from build123d import *

# Parameters (mm, degrees)
SKETCH1_R           = 100
BOSS_EXTRUDE1_DEPTH = 325
SKETCH2_R           = 181.25545507
SKETCH2_R_2         = 10
BOSS_EXTRUDE2_DEPTH = 5
FILLET1_R           = 20
BOSS_EXTRUDE3_DEPTH = 5


with BuildPart() as part:
    # Sketch1 → Boss-Extrude1 (new, symmetric)
    with BuildSketch(Plane(origin=(0, 0, 0), x_dir=(1, 0, 0), z_dir=(0, 1, 0))):
        with Locations(Location((0, 0, 0), (0, 0, 270))):
            Circle(SKETCH1_R)
    extrude(amount=BOSS_EXTRUDE1_DEPTH, both=True)

    # Sketch2 → Boss-Extrude2 (add, symmetric)
    with BuildSketch(Plane.XZ.offset(325)):
        with Locations(Location((0, 0, 0), (0, 0, 270))):
            Circle(SKETCH2_R)
        with Locations(Location((0, 147.291814794, 0), (0, 0, 270))):
            Circle(SKETCH2_R_2, mode=Mode.SUBTRACT)
        with Locations(Location((127.558453381, 73.645907397, 0), (0, 0, 270))):
            Circle(SKETCH2_R_2, mode=Mode.SUBTRACT)
        with Locations(Location((127.558453381, -73.645907397, 0), (0, 0, 270))):
            Circle(SKETCH2_R_2, mode=Mode.SUBTRACT)
        with Locations(Location((0, -147.291814794, 0), (0, 0, 270))):
            Circle(SKETCH2_R_2, mode=Mode.SUBTRACT)
        with Locations(Location((-127.558453381, -73.645907397, 0), (0, 0, 270))):
            Circle(SKETCH2_R_2, mode=Mode.SUBTRACT)
        with Locations(Location((-127.558453381, 73.645907397, 0), (0, 0, 270))):
            Circle(SKETCH2_R_2, mode=Mode.SUBTRACT)
    extrude(amount=BOSS_EXTRUDE2_DEPTH, both=True)

    # Fillet1
    fillet1_edges = [part.edges().sort_by_distance(p)[0] for p in [
        (0, -320, -100),
    ]]
    fillet(fillet1_edges, radius=FILLET1_R)

    # Sketch3 → Boss-Extrude3 (add, symmetric)
    with BuildSketch(Plane(origin=(0, 325, 0), x_dir=(1, 0, 0), z_dir=(0, 1, 0))):
        with BuildLine():
            Line((-90.193970518, -100.193970518), (90.193970518, -100.193970518))
            ThreePointArc((90.193970518, -100.193970518), (97.265038329, -97.265038329), (100.193970518, -90.193970518))
            Line((100.193970518, -90.193970518), (100.193970518, 90.193970518))
            ThreePointArc((100.193970518, 90.193970518), (97.265038329, 97.265038329), (90.193970518, 100.193970518))
            Line((90.193970518, 100.193970518), (-90.193970518, 100.193970518))
            ThreePointArc((-90.193970518, 100.193970518), (-97.265038329, 97.265038329), (-100.193970518, 90.193970518))
            Line((-100.193970518, 90.193970518), (-100.193970518, -90.193970518))
            ThreePointArc((-100.193970518, -90.193970518), (-97.265038329, -97.265038329), (-90.193970518, -100.193970518))
        make_face()
    extrude(amount=BOSS_EXTRUDE3_DEPTH, both=True)


solid = part.part
Could you check a few things on this model? Use its own coordinates, in mm. A direction names the side the tool comes from. Coordinates: 2 decimals unless noted, no trailing zeros. Write each loop counter-clockwise with the first axis right and the second up, starting at its lowest first coordinate (ties: lowest second). Pieces come first, ordered by that corner, then holes. Notation, with made-up numbers: (14.5, 39) - (59.5, 39) arc R20 cw to (59.5, 69) - close; hole circle Ø6 at (-30, 16). An arc over 180 degrees is marked (long way). Put each result on its own line as item: value. Start each with the question number.
Q1. I'm going to push flat-ended pins straight in: P1, Ø3, axis at y = 326.5, z = -35.5, coming from the -X side; P2, Ø1, axis at y = -258.5, z = 5, coming from the +X side; P3, Ø5, axis at y = 325, z = -6, coming from the +X side. Where does each tip first touch, or does it pass through?
Q2. I want a section at B-B on z = 0. Write out the boundary of the cut face in (x, y), plus the area to 3 significant figures.
Q3. I want a section at C-C on y = 171. Write out the boundary of the cut face in (x, z).
Q4. Which directions (+Z, -Z, +X, -X, +Y, -Y) give clear straight access to the entire face, cutting with the end or side of a thin tool? Please do faces 5 (the cylindrical face through (-3.83, -324.93, 138.054)), 6 (the flat face through (-45, 320, -90)).
Q5. I want a section at A-A on x = 0. Write out the boundary of the cut face in (y, z), plus the area to 3 significant figures.
Q6. Please list where these lines run through material, in increasing order: L1, parallel to Y at x = 90.5, z = -84; L2, parallel to Y at x = -95, z = 106; L3, parallel to Z at x = 3, y = 97.5.
Q7. Thinking about a two-plate mould opening in Z: for faces 1 (the flat face through (-118, -320, -38)), 2 (the cylindrical face through (-120.8, -324.93, -66.275)), 3 (the cylindrical face through (121.5, -324.9, 81.6)), 4 (the cylindrical face through (30.04, 14.34, 95.38)), which applies, pulls with the +Z half, pulls with the -Z half, needs draft (parallel to the pull), parting line crosses it, or undercut?
Q8. I want a section at D-D on x = 149.5. Write out the boundary of the cut face in (y, z).
Checks:
1. P1: x = -100.19
1. P2: x = 99.9
1. P3: x = 100.19
2. outline: (-181.26, -330) - (181.26, -330) - (181.26, -320) - (120, -320) arc R20 cw to (100, -300) - (100, 320) - (100.19, 320) - (100.19, 330) - (-100.19, 330) - (-100.19, 320) - (-100, 320) - (-100, -300) arc R20 cw to (-120, -320) - (-181.26, -320) - close
2. area: 134,000 mm²
3. outline: circle Ø200 at (0, 0)
4. face 5: +Y, -Y
4. face 6: none
5. outline: (-330, -181.26) - (-320, -181.26) - (-320, -157.29) - (-330, -157.29) - close; (-330, -137.29) - (-320, -137.29) - (-320, -120) arc R20 cw to (-300, -100) - (320, -100) - (320, -100.19) - (330, -100.19) - (330, 100.19) - (320, 100.19) - (320, 100) - (-300, 100) arc R20 cw to (-320, 120) - (-320, 137.29) - (-330, 137.29) - close; (-330, 157.29) - (-320, 157.29) - (-320, 181.26) - (-330, 181.26) - close
5. area: 133,000 mm²
6. L1: -330 to -320, 320 to 330
6. L2: -330 to -320
6. L3: -99.95 to 99.95
7. face 1: needs draft
7. face 2: undercut
7. face 3: undercut
7. face 4: parting line crosses it
8. outline: (-330, -102.49) - (-320, -102.49) - (-320, 102.49) - (-330, 102.49) - close
